Geometry: final body of the model. Coordinates: model frame, mm. A direction names the side the tool comes from. Round coordinates to 2 decimals unless told otherwise and drop trailing zeros. Order: outer loops, then holes, each group sorted by start corner. A loop starts at its lowest first (then second) coordinate and runs counter-clockwise, first axis right, second up. Notation, with made-up numbers: M 41.25,-7.75 L 47.25,-7.75 A26 ccw 47.25,27.25 Z; hole C 42,43.25 d7. An arc over 180 degrees is marked long. Put each result on its own line as item: value. Start each with the question number.
1) Access query for faces 1 (the flat face through (-12.065, 1, -2)), 2 (the flat face through (-22.52, 1.96, -9.78)), 3 (the cylindrical face through (-14.6, 3.35, -15.26)), 4 (the cylindrical face through (-15.742, 1.528, -3.835)). Directions: +Z, -Z, +X, -X, +Y, -Y. A direction counts if a zero-diameter tool reaches every point of the face in a straight line with its end or side. Return the directions, or none.
2) Section C-C, the plane y = 2.75. Return loops of the section in (x, z) (1 decimal), then the cut area to 3 significant figures.
3) First-contact query: P1, Ø1.5, axis at x = -19.5, z = -16, coming from the +Y side; P2, Ø0.6, axis at y = 3.5, z = -8, coming from the +X side; P3, Ø1.5, axis at x = -18.5, y = 3, coming from the -Z side; P4, Ø2, axis at y = 1.5, z = -7, coming from the +X side. Flat tips, straight axial feed; report the tip coordinate or a pass-through.
4) Draft query along Z for faces 5 (the cylindrical face through (-15.79, 1.53, -15.88)), 6 (the flat face through (-15, 3.6, -4)), 7 (the flat face through (-22.307, 1.192, -14.566)). Return one class per face: pulls with the +Z half, pulls with the -Z half, needs draft (parallel to the pull), parting line crosses it, or undercut.
5) Material intervals for probe 1 along Z at (x, y) = (-17.5, 1.9); probe 2 along Z at (x, y) = (-15.5, 2.45); probe 3 along X at (y, z) = (0.3, -4.75), sorted ascending. Write a range as [from, to].
6) Section B-B, the plane x = -16.75. Return loops of the section in (y, z), then the cut area to 3 significant figures.
7) Section D-D, the plane z = -5.25. Return loops of the section in (x, y).
8) Section A-A, the plane z = -12.25. Return loops of the section in (x, y).
Autodesk Inventor part; units mm, degrees
ref_plane "Arbeitsebene4" through (-11.5157, 3.1, -14.361) normal (1, 0, 0) x (0, 0, -1)
ref_plane "Arbeitsebene5" through (-59.9023, 0, -9.9345) normal (0, 0, 1) x (0, 1, 0)
ref_plane "Arbeitsebene6" through (-17.4719, 3.6, -12.113) normal (-0.309, 0.9511, 0) x (0, 0, -1)
sketch "Skizze1" plane through (0, 0, 0) normal (0, 1, 0) x (-1, 0, 0)
  line L0 (0, 0) -> (21.4435, 0) construction
  line L1 (21.4435, 0) -> (21.4435, -17.7713) construction
  line L2 (21.4435, -17.7713) -> (0, -17.7713) construction
  line L3 (0, -17.7713) -> (0, 0) construction
  arc A0 (3.4429, -6.1124) -> (3.5369, -12.2987) centre (13.9264, -9.047) ccw
  arc A1 (3.5369, -12.2987) -> (17.7561, -12.2571) centre (10.6298, -6.5721) ccw
  arc A2 (17.8481, -6.152) -> (3.4429, -6.1124) centre (10.6298, -11.844) ccw
  arc A3 (17.7561, -12.2571) -> (17.8481, -6.152) centre (7.348, -9.047) ccw
  line L4 (3.0399, -9.047) -> (18.2399, -9.047)
  line L5 (10.6298, -2.6515) -> (10.6298, -15.6882)
  dimension "d9" = 15.2
  dimension "d12" = 13.0368
sketch "Skizze2" plane through (0, 0, 0) normal (0, 1, 0) x (-1, 0, 0)
  line L0 (0, 0) -> (21.0912, 0) construction
  line L1 (21.0912, 0) -> (21.0912, -24.0698) construction
  line L2 (21.0912, -24.0698) -> (0, -24.0698) construction
  line L3 (0, -24.0698) -> (0, 0) construction
  line L4 (17.3479, -12.3442) -> (17.5564, -17.8355)
  line L5 (0, -15.4153) -> (21.0912, -15.022)
  point P0 (17.4522, -15.0899)
  point P1 (17.8576, -15.0823)
  point P2 (2.6602, -15.3657)
  point P3 (10.1167, -10.9016)
  point P4 (10.0352, -15.2282)
  point P5 (10.3203, -19.614)
  point P6 (15.9484, -15.1179)
  point P7 (4.4034, -15.3332)
  dimension "d38" = 15.2
  dimension "d47" = 8.7147
sketch "Skizze3" plane through (0, 0, 0) normal (0, 1, 0) x (-1, 0, 0)
  line L0 (0, 0) -> (41.0457, 0) construction
  line L1 (41.0457, 0) -> (41.0457, -50.0176) construction
  line L2 (41.0457, -50.0176) -> (0, -50.0176) construction
  line L3 (0, -50.0176) -> (0, 0) construction
  arc A0 (26.8609, -29.1094) -> (14.9484, -29.1094) centre (20.9046, -43.0907) ccw
  arc A1 (14.9484, -37.9624) -> (26.8609, -37.9624) centre (20.9046, -23.981) ccw
  line L4 (26.8609, -29.1094) -> (26.8609, -37.9624)
  line L5 (14.9484, -37.9624) -> (14.9484, -29.1094)
  point P0 (20.7813, -28.8717)
  point P1 (20.996, -37.5841)
  dimension "d9" = 15.2
  dimension "d12" = 13.0368
  dimension "d49" = 8.715
  dimension "d57" = 15.1972
  dimension "d58" = 15.1972
  dimension "d59" = 11.9125
  dimension "d67" = 8.853
  dimension "d69" = 0
  dimension "d70" = 8.853
sketch "Skizze4" plane through (0, 0, 0) normal (0, 1, 0) x (-1, 0, 0)
  arc A0 (19.2206, -6.6251) -> (3.7078, -6.5825) centre (11.4473, -12.755) ccw
  arc A1 (19.1216, -13.1996) -> (19.2206, -6.6251) centre (7.9131, -9.7427) ccw
  arc A2 (3.8091, -13.2445) -> (19.1216, -13.1996) centre (11.4473, -7.0776) ccw
  arc A3 (3.7078, -6.5825) -> (3.8091, -13.2445) centre (14.9974, -9.7427) ccw
  arc A4 (20.1996, -6.1308) -> (2.731, -6.0835) centre (11.4473, -12.755) ccw
  arc A5 (20.0894, -13.7103) -> (20.1996, -6.1308) centre (7.9131, -9.7427) ccw
  arc A6 (2.8436, -13.7601) -> (20.0894, -13.7103) centre (11.4473, -7.0776) ccw
  arc A7 (2.731, -6.0835) -> (2.8436, -13.7601) centre (14.9974, -9.7427) ccw
  point P0 (0, 0)
  dimension "d60" = 1.077
extrude "Extrusion1" add sketch "Skizze4" along normal blind 3.1
sketch "Skizze8" plane through (0, 3.1, 0) normal (0, 1, 0) x (1, 0, 0)
  line L0 (-17.4719, 5.508) -> (-17.4719, 14.361)
  arc A0 (-17.4719, 5.508) -> (-5.5595, 5.508) centre (-11.5157, 19.4893) ccw
  arc A1 (-5.5595, 14.361) -> (-17.4719, 14.361) centre (-11.5157, 0.3796) ccw
  line L1 (-5.5595, 14.361) -> (-5.5595, 5.508)
  line L2 (-17.4719, 5.508) -> (-5.5595, 14.361) construction
  line L3 (-17.4719, 14.361) -> (-5.5595, 5.508) construction
  arc A2 (-19.1216, 13.1996) -> (-19.2206, 6.6251) centre (-7.9131, 9.7427) ccw construction
  arc A3 (-3.8091, 13.2445) -> (-19.1216, 13.1996) centre (-11.4473, 7.0776) ccw construction
  arc A4 (-3.7078, 6.5825) -> (-3.8091, 13.2445) centre (-14.9974, 9.7427) ccw construction
  arc A5 (-19.2206, 6.6251) -> (-3.7078, 6.5825) centre (-11.4473, 12.755) ccw construction
  arc A6 (-20.1996, 6.1308) -> (-2.731, 6.0835) centre (-11.4473, 12.755) ccw
  arc A7 (-2.731, 6.0835) -> (-2.8436, 13.7601) centre (-14.9974, 9.7427) ccw
  arc A8 (-2.8436, 13.7601) -> (-20.0894, 13.7103) centre (-11.4473, 7.0776) ccw
  arc A9 (-20.0894, 13.7103) -> (-20.1996, 6.1308) centre (-7.9131, 9.7427) ccw
  line L4 (-19.2206, 6.6251) -> (-3.8091, 13.2445) construction
  line L5 (-19.1216, 13.1996) -> (-3.7078, 6.5825) construction
  point P0 (0, 0)
  point P1 (-11.5157, 9.9345)
  point P2 (-11.5157, 9.9345)
extrude "Extrusion3" add sketch "Skizze8" along normal blind 0.5
sketch "Skizze9" plane through (0, 0, 0) normal (0, 0, 1) x (1, 0, 0)
  line L0 (-2.731, 0) -> (-20.1996, 0) construction
  line L1 (-2.731, 0) -> (-2.731, 3.6) construction
  line L2 (-20.1996, 3.6) -> (-2.731, 3.6) construction
  line L3 (-20.1996, 0) -> (-20.1996, 3.6) construction
  line L4 (-3.8091, 0) -> (-19.1216, 0)
  line L5 (-11.4653, 0) -> (-12.0653, 0)
  line L6 (-12.0653, 0) -> (-12.0653, 1.55)
  arc A0 (-11.4653, 2.15) -> (-12.0653, 1.55) centre (-11.4653, 1.55) ccw
  line L7 (-11.4653, 1.55) -> (-11.4653, 2.15) construction
  line L8 (-11.4653, 1.55) -> (-12.0653, 1.55) construction
  line L9 (-11.4653, 0) -> (-11.4653, 6.3928) construction
  line L10 (-20.1996, 0) -> (-2.731, 0) construction
  line L11 (-10.8653, 0) -> (-10.8653, 1.55)
  arc A1 (-10.8653, 1.55) -> (-11.4653, 2.15) centre (-11.4653, 1.55) ccw
  line L12 (-11.4653, 0) -> (-10.8653, 0)
  point P0 (0, 0)
  dimension "d75" = 0.6
  dimension "d76" = 90
  dimension "d77" = 1.55
extrude "Extrusion4" cut sketch "Skizze9" against normal up to next
sketch "Skizze10" plane through (0, 0, 0) normal (0, 1, 0) x (-1, 0, 0)
  arc A0 (5.5595, -14.361) -> (17.4719, -14.361) centre (11.5157, -0.3796) ccw
  line L0 (5.5595, -14.361) -> (5.5595, -5.508)
  arc A1 (17.4719, -5.508) -> (5.5595, -5.508) centre (11.5157, -19.4893) ccw
  line L1 (17.4719, -5.508) -> (17.4719, -14.361)
  arc A2 (20.1996, -6.1308) -> (2.731, -6.0835) centre (11.4473, -12.755) ccw
  arc A3 (2.731, -6.0835) -> (2.8436, -13.7601) centre (14.9974, -9.7427) ccw
  arc A4 (2.8436, -13.7601) -> (20.0894, -13.7103) centre (11.4473, -7.0776) ccw
  arc A5 (20.0894, -13.7103) -> (20.1996, -6.1308) centre (7.9131, -9.7427) ccw
  arc A6 (20.1996, -6.1308) -> (2.731, -6.0835) centre (11.4473, -12.755) ccw
  line L2 (5.5595, -14.361) -> (5.5595, -5.508) construction
  line L3 (5.5595, -9.9345) -> (-7.2798, -9.9345) construction
  line L4 (3.7452, -4.9345) -> (-3.2387, -5.9345)
  line L5 (-3.2387, -5.9345) -> (-3.2387, -9.9345)
  line L6 (3.9282, -14.9607) -> (-3.2387, -13.9345)
  line L7 (-3.2387, -13.9345) -> (-3.2387, -9.9345)
  line L8 (17.4719, -5.508) -> (17.4719, -14.361) construction
  line L9 (17.4719, -9.9345) -> (23.9782, -9.9345) construction
  line L10 (22.5662, -4.9105) -> (14.2748, -4.9105) construction
  arc A7 (2.731, -6.0835) -> (2.8436, -13.7601) centre (14.9974, -9.7427) ccw construction
  line L11 (27.4359, -9.9345) -> (27.4359, -5.9345)
  line L12 (27.4359, -5.9345) -> (19.125, -4.9105)
  line L13 (27.4359, -9.9345) -> (27.4359, -13.9345)
  line L14 (27.4359, -13.9345) -> (18.9455, -14.9805)
  point P0 (0, 0)
  point P1 (3.7452, -14.9345)
  point P2 (2.1983, -9.9345)
  point P3 (2.1983, -9.9345)
  point P4 (19.125, -14.9584)
  dimension "d80" = 5
  dimension "d82" = 8.7982
  dimension "d84" = 4
  dimension "d85" = 4
  dimension "d112" = 10.07
  dimension "d116" = 9.964
extrude "Extrusion5" add sketch "Skizze10" along normal up to surface (3.6 mm away) contours A2 L12 L11 L13 L14 A4 A5 | A2 A3 A4 L6 L7 L5 L4
ref_plane "Arbeitsebene4" through (-11.5157, 3.1, -14.361) normal (1, 0, 0) x (0, 0, -1)
split "Trennen4" plane through (-11.5157, 3.1, -14.361) removes the side toward (1, 0, 0)
ref_plane "Arbeitsebene5" through (-59.9023, 0, -9.9345) normal (0, 0, 1) x (0, 1, 0)
ref_plane "Arbeitsebene6" through (-17.4719, 3.6, -12.113) normal (-0.309, 0.9511, 0) x (0, 0, -1)
split "Trennen5" plane through (-17.4719, 3.6, -12.113) removes the side toward (-0.309, 0.9511, 0)
sketch "Skizze13" plane through (0, 0, 0) normal (0, -1, 0) x (1, 0, 0)
  line L0 (-3.7452, -4.9345) -> (3.2387, -5.9345)
  line L1 (3.2387, -13.9345) -> (-3.9282, -14.9607)
  arc A0 (-3.8091, -13.2445) -> (-3.7078, -6.5825) centre (-14.9974, -9.7427) ccw
  arc A1 (-3.3813, -14.9345) -> (-2.5876, -6.9345) centre (-14.9974, -9.7427) ccw
  line L2 (3.2387, -5.9345) -> (3.2387, -13.9345)
  line L3 (3.2387, -6.9345) -> (-2.5876, -6.9345)
  line L4 (3.2387, -14.9345) -> (-3.3813, -14.9345)
  point P0 (0, 0)
  dimension "d92" = 1
  dimension "d104" = 1
  dimension "d105" = 1
sketch "Skizze12" plane through (0, 0, 0) normal (0, -1, 0) x (1, 0, 0)
  arc A0 (-3.5369, -12.2987) -> (-3.4429, -6.1124) centre (-13.9264, -9.047) ccw
  arc A1 (-17.7561, -12.2571) -> (-3.5369, -12.2987) centre (-10.6298, -6.5721) ccw
  arc A2 (-17.8481, -6.152) -> (-17.7561, -12.2571) centre (-7.348, -9.047) ccw
  arc A3 (-11.2465, -2.6722) -> (-17.8481, -6.152) centre (-10.6298, -11.844) ccw
  line L0 (-11.2465, -2.6722) -> (-11.2465, -1.6701)
  arc A4 (-11.2465, -1.6701) -> (-17.9952, -4.7985) centre (-10.6298, -11.844) ccw
  line L1 (-25.4478, -5.693) -> (-17.9952, -4.7985)
  line L2 (-25.4478, -12.757) -> (-25.4478, -5.693)
  line L3 (-17.8374, -13.6705) -> (-25.4478, -12.757)
  arc A5 (-17.8374, -13.6705) -> (-3.4226, -13.6708) centre (-10.6298, -6.5721) ccw
  line L4 (-17.9952, -4.7985) -> (-17.963, -6.6068)
  line L5 (-17.8695, -11.8632) -> (-17.8374, -13.6705)
  arc A6 (-2.3529, -11.757) -> (-2.2753, -6.693) centre (-13.9264, -9.047) ccw
  line L6 (4.0611, -5.693) -> (4.0611, -6.693)
  line L7 (-3.2644, -4.7985) -> (4.0611, -5.693)
  arc A7 (-3.2644, -4.7985) -> (-10.0465, -1.6682) centre (-10.6298, -11.844) ccw
  line L8 (-10.0465, -1.6682) -> (-10.0465, -2.67)
  arc A8 (-3.4429, -6.1124) -> (-10.0465, -2.67) centre (-10.6298, -11.844) ccw
  line L9 (4.0611, -12.757) -> (-3.4226, -13.6708)
  line L10 (4.0611, -11.757) -> (4.0611, -12.757)
  line L11 (4.0611, -11.757) -> (-2.3529, -11.757)
  line L12 (-2.2753, -6.693) -> (4.0611, -6.693)
  point P0 (0, 0)
properties part number "Main_afterRhino_V2" material "Gold"
Result sheet:
1. face 1: +Z, +X, -Y
1. face 2: +Z, -Z, -X, +Y
1. face 3: +X, +Y, -Y
1. face 4: +X, -Y
2. outline: M -20.1,-14.8 L -18.9,-15 A10.9 ccw -11.5,-18 L -11.5,-16.9 A9.8 cw -19.1,-13.2 A11.7 cw -19.2,-6.6 A9.9 cw -11.5,-2.9 L -11.5,-1.8 A11 ccw -19.1,-4.9 L -20.1,-5 Z
2. area: 25.7 mm2
3. P1: passes through
3. P2: stops at x = -17.47
3. P3: stops at z = -15.96
3. P4: stops at x = -18.68
4. face 5: undercut
4. face 6: needs draft
4. face 7: pulls with the -Z half
5. probe 1: z = [-16.14, -14.81], [-4.92, -3.6]
5. probe 2: z = [-17.19, -16.02], [-3.72, -2.55]
5. probe 3: x = [-18.96, -17.27]
6. outline: M 0,-16.59 L 3.6,-16.59 L 3.6,-14.65 L 3.1,-14.65 L 3.1,-15.34 L 0,-15.34 Z; M 0,-4.4 L 3.1,-4.4 L 3.1,-5.22 L 3.6,-5.22 L 3.6,-3.14 L 0,-3.14 Z
6. area: 9.78 mm2
7. outline: M -21.88,0 L -17.9,0 L -17.9,3.1 L -16.83,3.1 L -16.83,3.6 L -17.47,3.6 L -21.88,2.17 Z
8. outline: M -27.44,0 L -19.37,0 L -19.37,2.98 L -27.44,0.36 Z; M -19.01,3.1 L -17.47,3.1 L -17.47,3.6 Z
